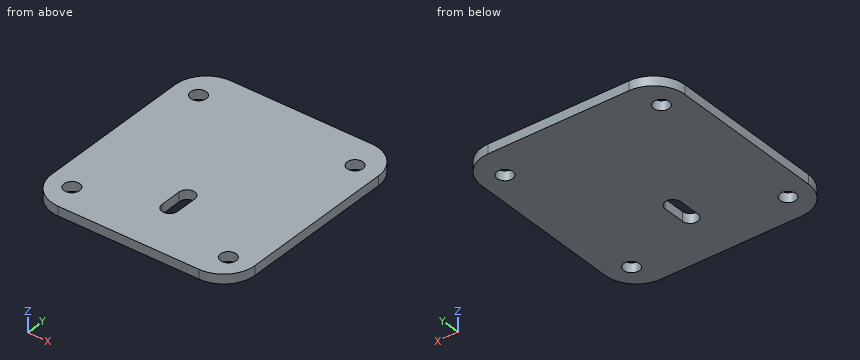
```python
from build123d import *

# Parameters (mm, degrees)
SKETCH1_R           = 2.5
BOSS_EXTRUDE1_DEPTH = 3
FILLET1_R           = 10
FILLET1_R_2         = 15
FILLET1_R_3         = 50
SKETCH2_R           = 1.75
SKETCH2_R_2         = 12
CUT_EXTRUDE1_DEPTH  = 82.389898264
SKETCH4_W           = 65
SKETCH4_H           = 34.30914122
CUT_EXTRUDE2_DEPTH  = 82.389898264
FILLET2_R           = 10
SKETCH5_R           = 2.5
CUT_EXTRUDE3_DEPTH  = 52.820000965


with BuildPart() as part:
    # Sketch1 → Boss-Extrude1 (new body)
    with BuildSketch(Plane.XY):
        Polygon((-32.5, 30), (32.5, 30), (32.5, -62.640754554), (0, -87.640754554), (-32.5, -62.640754554), align=None)
        with Locations((25, 20)):
            Circle(SKETCH1_R, mode=Mode.SUBTRACT)
        with Locations((-25, 20)):
            Circle(SKETCH1_R, mode=Mode.SUBTRACT)
        with BuildLine():
            Line((2.5, -16.5), (2.5, -23.5))
            ThreePointArc((2.5, -23.5), (0, -26), (-2.5, -23.5))
            Line((-2.5, -23.5), (-2.5, -16.5))
            ThreePointArc((-2.5, -16.5), (0, -14), (2.5, -16.5))
        make_face(mode=Mode.SUBTRACT)
    extrude(amount=BOSS_EXTRUDE1_DEPTH)

    # Fillet1
    # the kernel refuses this fillet: 50, 15, 10 mm, written as the material it takes off along each edge
    with BuildSketch(Plane(origin=(32.5, 30, -25), x_dir=(-1, 0, 0), z_dir=(0, 0, 1))) as fillet1_piece_1:
        with BuildLine():
            CenterArc((FILLET1_R, FILLET1_R), FILLET1_R, 180, 90)
            Line((0, FILLET1_R), (0, 0))
            Line((0, 0), (FILLET1_R, 0))
        make_face()
    extrude(amount=53, mode=Mode.SUBTRACT)
    with BuildSketch(Plane(origin=(-32.5, 30, -25), x_dir=(1, 0, 0), z_dir=(0, 0, 1))) as fillet1_piece_2:
        with BuildLine():
            CenterArc((FILLET1_R, -FILLET1_R), FILLET1_R, 90, 90)
            Line((0, -FILLET1_R), (0, 0))
            Line((0, 0), (FILLET1_R, 0))
        make_face()
    extrude(amount=53, mode=Mode.SUBTRACT)
    with BuildSketch(Plane(origin=(-32.5, -62.640754554, -18.465056154), x_dir=(0.7926239891046004, -0.6097107608496921, 0), z_dir=(0, 0, 1)), Plane(origin=(32.5, -62.640754554, -18.465056154), x_dir=(0, 1, 0), z_dir=(0, 0, 1))) as fillet1_piece_3:
        with BuildLine():
            CenterArc((FILLET1_R_2 * 0.492401497451, FILLET1_R_2), FILLET1_R_2, 217.568592029, 52.431407971)
            Line((-FILLET1_R_2 * 0.300222491654, FILLET1_R_2 * 0.39028923915), (0, 0))
            Line((0, 0), (FILLET1_R_2 * 0.492401497451, 0))
        make_face()
    extrude(amount=39.930112309, mode=Mode.SUBTRACT)
    with BuildSketch(Plane(origin=(0, -87.640754554, -96.153846154), x_dir=(0.7926239891046001, 0.6097107608496922, 0), z_dir=(0, 0, 1))) as fillet1_piece_4:
        with BuildLine():
            CenterArc((FILLET1_R_3 * 0.769230769231, FILLET1_R_3), FILLET1_R_3, 194.862815942, 75.137184058)
            Line((-FILLET1_R_3 * 0.197311981699, FILLET1_R_3 * 0.743494423792), (0, 0))
            Line((0, 0), (FILLET1_R_3 * 0.769230769231, 0))
        make_face()
    extrude(amount=195.307692308, mode=Mode.SUBTRACT)

    # Sketch2 → Cut-Extrude1 (cut, through all)
    with BuildSketch(Plane.XY.offset(3)):
        with Locations((12, -42)):
            Circle(SKETCH2_R)
        with Locations((-12, -42)):
            Circle(SKETCH2_R)
        with Locations((-12, -66)):
            Circle(SKETCH2_R)
        with Locations((12, -66)):
            Circle(SKETCH2_R)
        with Locations((0, -54)):
            Circle(SKETCH2_R_2)
    extrude(amount=-CUT_EXTRUDE1_DEPTH, mode=Mode.SUBTRACT)

    # Sketch4 → Cut-Extrude2 (cut, through all)
    with BuildSketch(Plane.XY.offset(3)):
        with Locations((0, -57.40457061)):
            Rectangle(SKETCH4_W, SKETCH4_H)
    extrude(amount=-CUT_EXTRUDE2_DEPTH, mode=Mode.SUBTRACT)

    # Fillet2
    fillet2_edges = [part.edges().sort_by_distance(p)[0] for p in [
        (-32.5, -40.25, 1.5),
        (32.5, -40.25, 1.5),
    ]]
    fillet(fillet2_edges, radius=FILLET2_R)

    # Sketch5 → Cut-Extrude3 (cut, through all)
    with BuildSketch(Plane.XY.offset(3)):
        with Locations((25, -31.5)):
            Circle(SKETCH5_R)
        with Locations(Location((-25, -31.5, 0), (0, 0, 180))):
            Circle(SKETCH5_R)
    extrude(amount=-CUT_EXTRUDE3_DEPTH, mode=Mode.SUBTRACT)


solid = part.part
```
Can you work these out from the model? Positions are in its coordinate system, mm. Round coordinates to 2 decimals unless told otherwise and drop trailing zeros. Loops run counter-clockwise (first coordinate to the right, second up) from the corner with the lowest first, then second, coordinate; pieces in that order, holes last.
Item 1: Suppose I cut it at A-A, the plane x = 0. Write out the boundary of the cut face in (y, z), then the cut area to 3 significant figures.
Item 2: Suppose I cut it at C-C, the plane y = -31.5. Write out the boundary of the cut face in (x, z).
Item 3: Please list where these lines run through material, in increasing order: L1, parallel to X at y = -20, z = 1.6; L2, parallel to Y at x = 25, z = 2.25; L3, parallel to X at y = 19, z = 2.35.
Item 4: Will these pins go through, and if not, where does the flat tip stop? pin 1 Ø3 at (x, y) = (25, 20) entering from -Z; pin 2 Ø1 at (y, z) = (21.5, 0.5) entering from +X; pin 3 Ø1.5 at (x, z) = (-24.5, 1) entering from -Y; pin 4 Ø8 at (x, y) = (19, -25.5) entering from -Z.
Item 5: Suppose I cut it at B-B, the plane z = 1.25. Write out the boundary of the cut face in (x, y), then the cut area to 3 significant figures.
Item 6: Suppose I cut it at D-D, the plane x = 25. Write out the boundary of the cut face in (y, z).
Reported:
1. outline: (-40.25, 0) - (-26, 0) - (-26, 3) - (-40.25, 3) - close; (-14, 0) - (30, 0) - (30, 3) - (-14, 3) - close
1. area: 175 mm2
2. outline: (-32.42, 0) - (-27.5, 0) - (-27.5, 3) - (-32.42, 3) - close; (-22.5, 0) - (22.5, 0) - (22.5, 3) - (-22.5, 3) - close; (27.5, 0) - (32.42, 0) - (32.42, 3) - (27.5, 3) - close
3. L1: x = -32.5 to -2.5, 2.5 to 32.5
3. L2: y = -39.93 to -34, -29 to 17.5, 22.5 to 29.68
3. L3: x = -32.5 to -27.29, -22.71 to 22.71, 27.29 to 32.5
4. pin 1: passes through
4. pin 2: stops at x = 32.45
4. pin 3: stops at y = -40.17
4. pin 4: stops at z = 0
5. outline: (-32.5, -30.25) arc R10 ccw to (-22.5, -40.25) - (22.5, -40.25) arc R10 ccw to (32.5, -30.25) - (32.5, 20) arc R10 ccw to (22.5, 30) - (-22.5, 30) arc R10 ccw to (-32.5, 20) - close; hole circle Ø5 at (-25, -31.5); hole circle Ø5 at (-25, 20); hole (-2.5, -23.5) arc R2.5 ccw to (2.5, -23.5) - (2.5, -16.5) arc R2.5 ccw to (-2.5, -16.5) - close; hole circle Ø5 at (25, -31.5); hole circle Ø5 at (25, 20)
5. area: 4,350 mm2
6. outline: (-39.93, 0) - (-34, 0) - (-34, 3) - (-39.93, 3) - close; (-29, 0) - (17.5, 0) - (17.5, 3) - (-29, 3) - close; (22.5, 0) - (29.68, 0) - (29.68, 3) - (22.5, 3) - close
